Geometry check sheet. Reference: the model listing, model coordinates, mm. A direction names the side the tool comes from. Coordinates: 2 decimals unless noted, no trailing zeros. Loops run counter-clockwise (first coordinate to the right, second up) from the corner with the lowest first, then second, coordinate; pieces in that order, holes last. Notation, with made-up numbers: M 63,82.5 L 69,82.5 A6 cw 69,91.5 Z; hole C 46,16 d1. An arc over 180 degrees is marked long. Use CSV: the item, a comma, the result in double quotes.
```python
from build123d import *

# Parameters (mm, degrees)
SKETCH1_R           = 1.5499999999999983
BOSS_EXTRUDE1_DEPTH = 2
CUT_EXTRUDE1_DEPTH  = 2
BOSS_EXTRUDE2_DEPTH = 12
SKETCH4_R           = 1.5000000000000009
CUT_EXTRUDE2_DEPTH  = 2
SKETCH_8_R          = 3
EXTRUDE_1_DEPTH     = 12
CHAMFER6_SIZE       = 3
SKETCH_1_R          = 4.0000000000000036
CUT_EXTRUDE_1_DEPTH = 10
SKETCH_9_R          = 1.5000000000000009
CUT_EXTRUDE_2_DEPTH = 125.68382559540109
FILLET_1_R          = 2
SKETCH_10_W         = 2
SKETCH_10_H         = 7.38673868931825
CUT_EXTRUDE_3_DEPTH = 1


with BuildPart() as part:
    # Sketch1 → Boss-Extrude1 (new body)
    with BuildSketch(Plane(origin=(0, 0, 0), x_dir=(0, 0, -1), z_dir=(1, 0, 0))):
        with BuildLine():
            Line((-25.968110327255765, 120.00000000000003), (25.968110327255765, 120.00000000000003))
            ThreePointArc((25.968110327255765, 120.00000000000003), (29.488419187011914, 79.62790655837495), (30.82293132778887, 39.124603227985936))
            ThreePointArc((30.82293132778887, 39.124603227985936), (29.206107258133628, 36.44471853371224), (26.083845229838534, 36.66239231138328))
            ThreePointArc((26.083845229838534, 36.66239231138328), (-6.3665e-13, 44.994421787238764), (-26.083845229839092, 36.66239231138189))
            ThreePointArc((-26.083845229839092, 36.66239231138189), (-29.20610725813421, 36.44471853371079), (-30.82293132778949, 39.1246032279845))
            ThreePointArc((-30.82293132778949, 39.1246032279845), (-29.488419187012596, 79.6279065583745), (-25.968110327255765, 120.00000000000003))
        make_face()
        with Locations((-11.999999999999995, 115)):
            Circle(SKETCH1_R, mode=Mode.SUBTRACT)
        with Locations((12.000000000000005, 115)):
            Circle(SKETCH1_R, mode=Mode.SUBTRACT)
    extrude(amount=BOSS_EXTRUDE1_DEPTH)

    # Sketch2 → Cut-Extrude1 (cut)
    with BuildSketch(Plane(origin=(2, 0, 0), x_dir=(0, 0, -1), z_dir=(1, 0, 0))):
        with BuildLine():
            Line((4, 89.70000000000002), (4.000000000000003, 81.7))
            ThreePointArc((4.000000000000003, 81.7), (1.16e-15, 77.7), (-4.000000000000001, 81.7))
            Line((-4.000000000000001, 81.7), (-4.0000000000000036, 89.70000000000002))
            ThreePointArc((-4.0000000000000036, 89.70000000000002), (-3.1e-16, 93.70000000000002), (4, 89.70000000000002))
        make_face()
    extrude(amount=-CUT_EXTRUDE1_DEPTH, mode=Mode.SUBTRACT)

    # Sketch3 → Boss-Extrude2 (add)
    with BuildSketch(Plane(origin=(2, 0, 0), x_dir=(0, 0, -1), z_dir=(1, 0, 0))):
        with BuildLine():
            Line((-21.94183683045926, 120.00000000000003), (-25.968110327255765, 120.00000000000003))
            ThreePointArc((-25.968110327255772, 120.00000000000003), (-29.488419187012482, 79.6279065583743), (-30.82293132778932, 39.124603227984586))
            ThreePointArc((-30.822931327789238, 39.1246032279846), (-29.56718535087633, 36.66600228940771), (-26.834368801169504, 36.274428235935545))
            ThreePointArc((-26.83436880116949, 36.27442823593551), (-25.56563052181184, 78.20602334586083), (-21.941836830459124, 120.00000000000003))
        make_face()
        with BuildLine():
            Line((25.968110327255545, 119.99999999999999), (21.941836830459355, 119.99999999999999))
            ThreePointArc((21.94183683045935, 120.00000000000006), (25.565630521812068, 78.20602334586118), (26.834368801169717, 36.27442823593619))
            ThreePointArc((26.834368801169717, 36.27442823593619), (29.567185350876464, 36.66600228940895), (30.822931327789195, 39.124603227985936))
            ThreePointArc((30.822931327789092, 39.124603227985936), (29.48841918701214, 79.62790655837497), (25.96811032725543, 119.99999999999999))
        make_face()
    extrude(amount=BOSS_EXTRUDE2_DEPTH)

    # Sketch4 → Cut-Extrude2 (cut)
    with BuildSketch(Plane.ZY):
        with Locations((-12, 48)):
            Circle(SKETCH4_R)
        with Locations((12, 48)):
            Circle(SKETCH4_R)
    extrude(amount=-CUT_EXTRUDE2_DEPTH, mode=Mode.SUBTRACT)

    # 草图8 → 凸台-拉伸1 (add)
    with BuildSketch(Plane(origin=(2, 0, 0), x_dir=(0, 0, -1), z_dir=(1, 0, 0))):
        with Locations(Location((-12, 48, 0), (0, 0, 180))):
            Circle(SKETCH_8_R)
        with Locations(Location((12, 48, 0), (0, 0, 180))):
            Circle(SKETCH_8_R)
    extrude(amount=EXTRUDE_1_DEPTH)

    # Chamfer6
    chamfer6_edges = [part.edges().sort_by_distance(p)[0] for p in [
        (2, 78.20602334586118, -25.565630521811954),
        (2, 78.20602334586081, 25.565630521811727),
    ]]
    chamfer(chamfer6_edges, length=CHAMFER6_SIZE)

    # 草图1 → 切除-拉伸1 (cut)
    with BuildSketch(Plane.ZY):
        with Locations((0, 110.00000000000003)):
            Circle(SKETCH_1_R)
    extrude(amount=-CUT_EXTRUDE_1_DEPTH, mode=Mode.SUBTRACT)

    # 草图9 → 切除-拉伸2 (cut, through all)
    with BuildSketch(Plane.ZY):
        with Locations((-12, 48)):
            Circle(SKETCH_9_R)
        with Locations((12, 48)):
            Circle(SKETCH_9_R)
    extrude(amount=-CUT_EXTRUDE_2_DEPTH, mode=Mode.SUBTRACT)

    # 圆角1
    fillet_1_edges = [part.edges().sort_by_distance(p)[0] for p in [
        (0, 44.994421787238764, 4.9916e-13),
        (0, 36.44471853371079, 29.20610725813421),
        (0, 79.62790655837429, 29.488419187012596),
        (0, 79.62790655837495, -29.4884191870118),
        (0, 36.44471853371224, -29.206107258133624),
    ]]
    fillet(fillet_1_edges, radius=FILLET_1_R - 0.0001)  # a hair under: the kernel refuses the full size

    # 草图10 → 切除-拉伸3 (cut)
    with BuildSketch(Plane.ZY):
        with Locations((0, 47.46265164885683)):
            Rectangle(SKETCH_10_W, SKETCH_10_H)
    extrude(amount=-CUT_EXTRUDE_3_DEPTH, mode=Mode.SUBTRACT)


solid = part.part
```
1. Gauge pin test, flat ends, axial feed: P1, Ø3, axis at y = 115, z = 12, coming from the -X side; P2, Ø4, axis at y = 115, z = -12, coming from the +X side; P3, Ø6, axis at x = 6.5, y = 60, coming from the -Z side; P4, Ø0.6, axis at x = 1, y = 87.5, coming from the +Z side. Record the tip position at first contact, or that the pin passes through.
The answers:
P1,"through"
P2,"x = 2"
P3,"z = -30.5"
P4,"z = 28.85"
2. Section check A-A, the plane x = 10.5. Record the cut outline in (y, z).
The answers:
outline,"M 36.27,-26.83 A3 ccw 39.12,-30.82 A750 ccw 120,-25.97 L 120,-21.94 A746 cw Z; M 36.27,26.83 A746 cw 120,21.94 L 120,25.97 A750 ccw 39.12,30.82 A3 ccw Z; C 48,-12 d6; C 48,12 d6; hole C 48,-12 d3; hole C 48,12 d3"
3. Set-up check for faces 1 (the cylindrical face through (1, 93.7, 0.1)), 2 (the cylindrical face through (8, 45, 12)), 3 (the conical face through (3.188, 78.86, -23.712)): record each of +Z, -Z, +X, -X, +Y, -Y from which the full face is reachable in a straight line by a thin tool's end or side.
The answers:
face 1,"+X, -X"
face 2,"+X"
face 3,"+X, -Y"
4. Thickness scan on line 1 (Y direction, x = 1.4, z = -12); line 2 (Z direction, x = 0.85, y = 115); line 3 (Y direction, x = 4.25, z = 12). Record the ranges inside material, lowest first. Write a range as [from, to].
The answers:
line 1,"[43.46, 46.5], [49.5, 113.45], [116.55, 120]"
line 2,"[-26.16, -13.55], [-10.45, 10.45], [13.55, 26.16]"
line 3,"[45, 46.5], [49.5, 51]"
5. Release check for a two-part mould opening along Z. For faces 4 (the cylindrical face through (9.4, 77.6, 25.6)), 5 (the cylindrical face through (7.916, 80.194, -29.454)), 6 (the flat face through (14, 79, 27)) record: +Z half, -Z half, draft (parallel to the pull), parting line (faces both ways), or undercut.
The answers:
face 4,"undercut"
face 5,"-Z half"
face 6,"draft"
6. Section check B-B, the plane z = 12. Count the separate pieces of the cut face and the enclosed holes in it, plus the area to 3 significant figures.
The answers:
separate pieces,"3"
enclosed holes,"0"
area,"176 mm^2"
